```python
from build123d import *

# Parameters (mm, degrees)
SKETCH1_W           = 30
SKETCH1_H           = 25
BOSS_EXTRUDE1_DEPTH = 2
SKETCH2_R           = 2
CUT_EXTRUDE1_DEPTH  = 2
SKETCH3_W           = 30
SKETCH3_H           = 2
BOSS_EXTRUDE3_DEPTH = 28
SKETCH4_R           = 2
CUT_EXTRUDE2_DEPTH  = 42.833001327


with BuildPart() as part:
    # Sketch1 → Boss-Extrude1 (new body)
    with BuildSketch(Plane.XY):
        Rectangle(SKETCH1_W, SKETCH1_H)
    extrude(amount=BOSS_EXTRUDE1_DEPTH)

    # Sketch2 → Cut-Extrude1 (cut)
    with BuildSketch(Plane.XY.offset(2)):
        with Locations((0, 2.5)):
            Circle(SKETCH2_R)
    extrude(amount=-CUT_EXTRUDE1_DEPTH, mode=Mode.SUBTRACT)

    # Sketch3 → Boss-Extrude3 (add)
    with BuildSketch(Plane.XY.offset(2)):
        with Locations((0, -11.5)):
            Rectangle(SKETCH3_W, SKETCH3_H)
    extrude(amount=BOSS_EXTRUDE3_DEPTH)

    # Sketch4 → Cut-Extrude2 (cut, through all)
    with BuildSketch(Plane.XZ.offset(12.5)):
        with Locations(Location((0, 20, 0), (0, 0, 270))):
            Circle(SKETCH4_R)
        with BuildLine():
            Line((-15, 30), (-15, 0))
            Line((-15, 0), (-10, 20))
            ThreePointArc((-10, 20), (-7.071067812, 27.071067812), (0, 30))
            Line((0, 30), (-15, 30))
        make_face()
        with BuildLine():
            Line((15, 30), (0, 30))
            ThreePointArc((0, 30), (7.071067812, 27.071067812), (10, 20))
            Line((10, 20), (15, 0))
            Line((15, 0), (15, 30))
        make_face()
    extrude(amount=-CUT_EXTRUDE2_DEPTH, mode=Mode.SUBTRACT)


solid = part.part
```
Can you work these out from the model? Positions are in its coordinate system, mm. A direction names the side the tool comes from. Give positions to 0.01 mm unless a question says otherwise; leave off trailing zeros. Loops run counter-clockwise (first coordinate to the right, second up) from the corner with the lowest first, then second, coordinate; pieces in that order, holes last. Notation, with made-up numbers: M -16,66.25 L 25,66.25 A31 ccw 25,94.25 Z; hole C 85,26 d2. An arc over 180 degrees is marked long. One line per question, with ' | ' between items. Start each with the question number.
Q1. If we mould it in two halves opening along Z, with no side actions, what happens to faces 1 (the flat face through (0, -12.5, 11)), 2 (the cylindrical face through (-1.2, -11.5, 21.6)), 3 (the flat face through (0, -1, 2))? For each: +Z half, -Z half, draft (parallel to the pull), parting line (faces both ways), or undercut.
Q2. If we section it at C-C (x = -8): Please give me the cut outline in (y, z), plus the area to 3 significant figures.
Q3. For faces 4 (the flat face through (14.7, -4.7, 1.2)), 5 (the flat face through (0, -10.5, 13)), which set-ups out of +Z, -Z, +X, -X, +Y, -Y let a thin tool reach every point of the face, with its end or its side?
Q4. For pin 1 Ø11.5 at (x, y) = (-7, 1.5) entering from +Z; pin 2 Ø3 at (x, y) = (-1.5, -4.5) entering from -Z; pin 3 Ø3 at (x, z) = (8.5, 4.5) entering from +Y, each with a flat end and sliding along its axis, tell me the tip position at first contact or that it passes through.
Q5. If we section it at A-A (y = 2.5): Please give me the cut outline in (x, z), plus the area to 3 significant figures.
Q6. If we section it at B-B (x = -1.5): Please give me the cut outline in (y, z), plus the area to 3 significant figures.
Q7. If I drill on line 1 (Y direction, x = 0, z = 1.35); line 2 (X direction, y = -11.55, z = 20); line 3 (Y direction, x = -4.75, z = 8.5), over which ranges is the centre line in solid material (lowest first)? Write a range as from..to.
Q8. If we section it at D-D (z = 13): Please give me the cut outline in (x, y).
Computed:
1) face 1: draft | face 2: undercut | face 3: +Z half
2) outline: M -12.5,0 L 12.5,0 L 12.5,2 L -10.5,2 L -10.5,26 L -12.5,26 Z | area: 98.0 mm²
3) face 4: +Z, +X, +Y, -Y | face 5: +Z, +X, -X, +Y
4) pin 1: stops at z = 2 | pin 2: stops at z = 0 | pin 3: stops at y = -10.5
5) outline: M -15,0 L -2,0 L -2,2 L -14.5,2 Z; M 2,0 L 15,0 L 14.5,2 L 2,2 Z | area: 51.0 mm²
6) outline: M -12.5,0 L 1.18,0 L 1.18,2 L -10.5,2 L -10.5,18.68 L -12.5,18.68 Z; M -12.5,21.32 L -10.5,21.32 L -10.5,29.89 L -12.5,29.89 Z; M 3.82,0 L 12.5,0 L 12.5,2 L 3.82,2 Z | area: 95.2 mm²
7) line 1: y = -12.5..0.5, 4.5..12.5 | line 2: x = -10..-2, 2..10 | line 3: y = -12.5..-10.5
8) outline: M -11.75,-12.5 L 11.75,-12.5 L 11.75,-10.5 L -11.75,-10.5 Z
